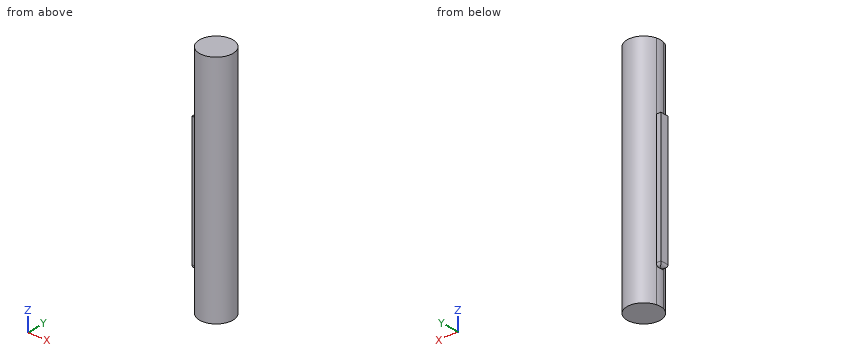
from build123d import *
from build123d.topology import SkipClean

# Parameters (mm, degrees)
BOSS_EXTRUDE1_DEPTH = 140
CUT_EXTRUDE1_DEPTH  = 20
CUT_EXTRUDE2_START  = -40
CUT_EXTRUDE2_DEPTH  = 40
CUT_EXTRUDE4_DEPTH  = 0.0001
FILLET2_SIZE        = 2


with BuildPart() as part:
    # Sketch1 → Boss-Extrude1 (new body)
    with BuildSketch(Plane(origin=(0, 0, 0), x_dir=(0, 1, 0), z_dir=(0, 0, 1))):
        with BuildLine():
            Line((-2.5, 12.5), (2.5, 12.5))
            Line((2.5, 12.5), (2.5, 9.682458))
            ThreePointArc((2.5, 9.682458), (0, -10), (-2.5, 9.682458))
            Line((-2.5, 9.682458), (-2.5, 12.5))
        make_face()
    extrude(amount=BOSS_EXTRUDE1_DEPTH)

    # Sketch2 → Cut-Extrude1 (cut)
    with SkipClean():  # the faces are left unmerged after this step: merging them gives an invalid solid
        with BuildSketch(Plane(origin=(0, 0, 0), x_dir=(1, 0, 0), z_dir=(0, 0, -1))):
            with BuildLine():
                Line((-9.682458, 2.5), (-12.5, 2.5))
                Line((-12.5, 2.5), (-12.5, -2.5))
                Line((-12.5, -2.5), (-9.682458, -2.5))
                ThreePointArc((-9.682458, -2.5), (-10, 0), (-9.682458, 2.5))
            make_face()
        extrude(amount=-CUT_EXTRUDE1_DEPTH, mode=Mode.SUBTRACT)

    # Sketch3 → Cut-Extrude2 (cut)
    with SkipClean():  # the faces are left unmerged after this step: merging them gives an invalid solid
        with BuildSketch(Plane.XY.offset(140).offset(CUT_EXTRUDE2_START)):
            with BuildLine():
                Line((-9.682458, 2.5), (-12.5, 2.5))
                Line((-12.5, 2.5), (-12.5, -2.5))
                Line((-12.5, -2.5), (-9.682458, -2.5))
                ThreePointArc((-9.682458, -2.5), (-10, 0), (-9.682458, 2.5))
            make_face()
        extrude(amount=CUT_EXTRUDE2_DEPTH, mode=Mode.SUBTRACT)

    # Sketch4 → Cut-Extrude4 (cut)
    with SkipClean():  # the faces are left unmerged after this step: merging them gives an invalid solid
        with BuildSketch(Plane(origin=(0, 0, 20), x_dir=(1, 0, 0), z_dir=(0, 0, -1))):
            with BuildLine():
                Line((-9.682458, 2.5), (-12.5, 2.5))
                Line((-12.5, 2.5), (-12.5, -2.5))
                Line((-12.5, -2.5), (-9.682458, -2.5))
                ThreePointArc((-9.682458, -2.5), (-10, 0), (-9.682458, 2.5))
            make_face()
        extrude(amount=-CUT_EXTRUDE4_DEPTH, mode=Mode.SUBTRACT)

    # Fillet2
    # a fillet whose section is not a circle: 2 mm, written as the material it takes off along each edge
    with BuildSketch(Plane(origin=(-4.682458, -2.5, 20.0001), x_dir=(0, 0, 1), z_dir=(-1, 0, 0))) as fillet2_piece_1_section:
        with BuildLine():
            Bezier((FILLET2_SIZE, 0), (0, 0), (0, FILLET2_SIZE), weights=[1, 1, 1])
            Line((0, FILLET2_SIZE), (0, 0))
            Line((0, 0), (FILLET2_SIZE, 0))
        make_face()
    fillet2_piece_1 = extrude(amount=12.817542, mode=Mode.PRIVATE)
    fillet2_piece_1 = fillet2_piece_1 - Plane(origin=(0, 0, 20.0001), x_dir=(-0.9682458365518543, 0.2500000000000001, 0), z_dir=(0, 0, -1)) * Cylinder(10, 34, mode=Mode.PRIVATE)
    add(fillet2_piece_1, mode=Mode.SUBTRACT)
    with BuildSketch(Plane(origin=(-17.5, 2.5, 20.0001), x_dir=(0, -1, 0), z_dir=(1, 0, 0))) as fillet2_piece_2_section:
        with BuildLine():
            Bezier((FILLET2_SIZE, 0), (0, 0), (0, -FILLET2_SIZE), weights=[1, 1, 1])
            Line((0, -FILLET2_SIZE), (0, 0))
            Line((0, 0), (FILLET2_SIZE, 0))
        make_face()
    fillet2_piece_2 = extrude(amount=12.817542, mode=Mode.PRIVATE)
    fillet2_piece_2 = fillet2_piece_2 - Plane(origin=(0, 0, 20.0001), x_dir=(-0.9682458365518561, 0.24999999999999276, 0), z_dir=(0, 0, -1)) * Cylinder(10, 34, mode=Mode.PRIVATE)
    add(fillet2_piece_2, mode=Mode.SUBTRACT)
    with BuildSketch(Plane(origin=(-12.5, -7.5, 20.0001), x_dir=(1, 0, 0), z_dir=(0, 1, 0))) as fillet2_piece_3:
        with BuildLine():
            Bezier((FILLET2_SIZE, 0), (0, 0), (0, -FILLET2_SIZE), weights=[1, 1, 1])
            Line((0, -FILLET2_SIZE), (0, 0))
            Line((0, 0), (FILLET2_SIZE, 0))
        make_face()
    extrude(amount=15, mode=Mode.SUBTRACT)


solid = part.part
Geometry check sheet. Reference: the model listing, model coordinates, mm. Round coordinates to 2 decimals unless told otherwise and drop trailing zeros. Write each loop counter-clockwise with the first axis right and the second up, starting at its lowest first coordinate (ties: lowest second). Pieces come first, ordered by that corner, then holes. Notation, with made-up numbers: (46.5, 36.25) - (103.5, 36.25) arc R17 cw to (103.5, 59.25) - close; hole circle Ø2 at (80.25, 7). An arc over 180 degrees is marked (long way). One line per item, written item: value.
1. Cross-section at C-C on z = 104. Record the boundary of the cut face in (x, y), and give its area (3 significant figures).
The answers:
outline: (-9.68, -2.5) arc R10 ccw (long way) to (-9.68, 2.5) arc R10 ccw to start
area: 314 mm^2
2. Cross-section at B-B on x = 5. Record the boundary of the cut face in (y, z), and give its area (3 significant figures).
The answers:
outline: (-8.66, 0) - (8.66, 0) - (8.66, 140) - (-8.66, 140) - close
area: 2,420 mm^2
3. Scan lines: L1, parallel to X at y = -0.75, z = 84; L2, parallel to Y at x = -0.75, z = 43.5; L3, parallel to Y at x = 6.5, z = 26. Record each from-to range of solid material in increasing order.
The answers:
L1: x = -12.5 to 9.97
L2: y = -9.97 to 9.97
L3: y = -7.6 to 7.6
4. Cross-section at A-A on z = 78. Record the boundary of the cut face in (x, y).
The answers:
outline: (-12.5, -2.5) - (-9.68, -2.5) arc R10 ccw (long way) to (-9.68, 2.5) - (-12.5, 2.5) - close
5. Depth check by flat-ended pin: pin 1 Ø3 at (x, y) = (-12, -1) entering from +Z; pin 2 Ø0.8 at (x, z) = (-11.5, 52.5) entering from +Y; pin 3 Ø2.5 at (x, z) = (-11.5, 77.5) entering from -Y. Enter the tip coordinate at first touch or a pass-through.
The answers:
pin 1: stops at z = 100
pin 2: stops at y = 2.5
pin 3: stops at y = -2.5
